Model file for the job. Use its own axes, mm. Face numbers are marked on the shaded views. A direction names the side the tool comes from. Round coordinates to 2 decimals unless told otherwise and drop trailing zeros. Write each loop counter-clockwise with the first axis right and the second up, starting at its lowest first coordinate (ties: lowest second). Pieces come first, ordered by that corner, then holes.
```python
from build123d import *

# Parameters (mm, degrees)
F0_W         = 50.8
F0_H         = 76.2
F1_DEPTH     = 6.35
F2_W         = 12.192
F2_H         = 25.4
F3_DEPTH     = 31.75
F5_D         = 12.7
F5_DEPTH     = 254
F5_TIP       = 3.8154649308
F6_R         = 12.69999
F7_T1_DEPTH  = 19.05001
F7_T3_DEPTH  = 76.2
F7_T5_DEPTH  = 38.1
F7_T7_DEPTH  = 38.1
F7_T9_DEPTH  = 2e-05
F7_T12_ANGLE = 90
F7_T14_ANGLE = 90
F7_T16_ANGLE = 90
F7_T18_ANGLE = 90
F7_T23_DEPTH = 31.75001
F7_T28_DEPTH = 38.1
F7_T35_DEPTH = 38.1
F7_T39_DEPTH = 31.75001
F7_T47_DEPTH = 38.1
F7_T51_DEPTH = 31.75001
F7_T59_DEPTH = 31.75001
F7_T64_DEPTH = 38.1


# Not quite as in the source:
# - a fillet or chamfer that OpenCascade refuses, or shapes differently, is made with other operations: its cross-section is extruded or revolved along the edge and cut away or added
# - a fillet or chamfer is up to 0.001 mm smaller than in the source, because OpenCascade refuses the exact size


with BuildPart() as f1:
    # F0 (on Top) → F1 (new body)
    with BuildSketch(Plane.XY):
        Rectangle(F0_W, F0_H)
    extrude(amount=F1_DEPTH)

    # F2 (on face) → F3 (join)
    with BuildSketch(Plane.XY.offset(6.35)):
        with Locations((-19.304, 0)):
            Rectangle(F2_W, F2_H)
        with Locations((19.304, 0)):
            Rectangle(F2_W, F2_H)
    extrude(amount=F3_DEPTH)

    # F5
    with Locations(Plane(origin=(-25.4, 0, 0), x_dir=(0, -1, 0), z_dir=(-1, 0, 0))):
        with Locations((0, 28.575)):
            Hole(F5_D / 2, depth=F5_DEPTH)
            with Locations((0, 0, -(F5_DEPTH + F5_TIP / 2))):  # 118° drill point
                Cone(0, F5_D / 2, F5_TIP, mode=Mode.SUBTRACT)

    # F6 (radius 12.7 in the source; OpenCascade refuses exactly that, so slightly less here)
    f6_edges = [f1.edges().sort_by_distance(p)[0] for p in [
        (19.304, 12.7, 38.1),
        (19.304, -12.7, 38.1),
        (-19.304, 12.7, 38.1),
        (-19.304, -12.7, 38.1),
    ]]
    fillet(f6_edges, radius=F6_R)

    # F7: fillet of radius 5.08 on 14 edges, made by hand

    # F7_s2 → F7_t1 (cut)
    with BuildSketch(Plane.XY.offset(6.35)):
        with BuildLine():
            ThreePointArc((-25.4, 7.62), (-23.9121024484, 11.2121024484), (-20.32, 12.7))
            Line((-20.32, 12.7), (-25.4, 12.7))
            Line((-25.4, 12.7), (-25.4, 7.62))
        make_face()
        with BuildLine():
            ThreePointArc((25.4, -7.62), (23.9121024484, -11.2121024484), (20.32, -12.7))
            Line((20.32, -12.7), (25.4, -12.7))
            Line((25.4, -12.7), (25.4, -7.62))
        make_face()
        with BuildLine():
            ThreePointArc((-25.4, -7.62), (-23.9121024484, -11.2121024484), (-20.32, -12.7))
            Line((-20.32, -12.7), (-25.4, -12.7))
            Line((-25.4, -12.7), (-25.4, -7.62))
        make_face()
        with BuildLine():
            ThreePointArc((25.4, 7.62), (23.9121024484, 11.2121024484), (20.32, 12.7))
            Line((20.32, 12.7), (25.4, 12.7))
            Line((25.4, 12.7), (25.4, 7.62))
        make_face()
    extrude(amount=F7_T1_DEPTH, mode=Mode.SUBTRACT)

    # F7_s4 → F7_t3 (cut)
    with BuildSketch(Plane.YZ.offset(-38.1)):
        with BuildLine():
            ThreePointArc((-33.02, 6.35), (-36.6121024484, 4.8621024484), (-38.1, 1.27))
            Line((-38.1, 1.27), (-38.1, 6.35))
            Line((-38.1, 6.35), (-33.02, 6.35))
        make_face()
        with BuildLine():
            ThreePointArc((33.02, 6.35), (36.6121024484, 4.8621024484), (38.1, 1.27))
            Line((38.1, 1.27), (38.1, 6.35))
            Line((38.1, 6.35), (33.02, 6.35))
        make_face()
    extrude(amount=F7_T3_DEPTH, mode=Mode.SUBTRACT)

    # F7_s6 → F7_t5 (cut)
    with BuildSketch(Plane.XZ.offset(12.7)):
        with BuildLine():
            ThreePointArc((20.32, 6.35), (23.9121024484, 4.8621024484), (25.4, 1.27))
            Line((25.4, 1.27), (25.4, 6.35))
            Line((25.4, 6.35), (20.32, 6.35))
        make_face()
        with BuildLine():
            ThreePointArc((-25.4, 1.27), (-23.9121024484, 4.8621024484), (-20.32, 6.35))
            Line((-20.32, 6.35), (-25.4, 6.35))
            Line((-25.4, 6.35), (-25.4, 1.27))
        make_face()
    extrude(amount=F7_T5_DEPTH, mode=Mode.SUBTRACT)

    # F7_s8 → F7_t7 (cut)
    with BuildSketch(Plane.XZ.offset(-50.8)):
        with BuildLine():
            ThreePointArc((20.32, 6.35), (23.9121024484, 4.8621024484), (25.4, 1.27))
            Line((25.4, 1.27), (25.4, 6.35))
            Line((25.4, 6.35), (20.32, 6.35))
        make_face()
        with BuildLine():
            ThreePointArc((-25.4, 1.27), (-23.9121024484, 4.8621024484), (-20.32, 6.35))
            Line((-20.32, 6.35), (-25.4, 6.35))
            Line((-25.4, 6.35), (-25.4, 1.27))
        make_face()
    extrude(amount=F7_T7_DEPTH, mode=Mode.SUBTRACT)

    # F7_s10 → F7_t9 (cut)
    with BuildSketch(Plane.XZ.offset(-1e-05)):
        with BuildLine():
            ThreePointArc((25.4, 33.02), (23.9121024484, 36.6121024484), (20.32, 38.1))
            Line((20.32, 38.1), (25.4, 38.1))
            Line((25.4, 38.1), (25.4, 33.02))
        make_face()
        with BuildLine():
            ThreePointArc((-25.4, 33.02), (-23.9121024484, 36.6121024484), (-20.32, 38.1))
            Line((-20.32, 38.1), (-25.4, 38.1))
            Line((-25.4, 38.1), (-25.4, 33.02))
        make_face()
    extrude(amount=F7_T9_DEPTH, mode=Mode.SUBTRACT)

    # F7_s11 → F7_t12 (revolve, cut)
    with BuildSketch(Plane.XY.offset(25.40001)):
        with BuildLine():
            ThreePointArc((-25.4, 7.62), (-23.9121024484, 11.2121024484), (-20.32, 12.7))
            Line((-20.32, 12.7), (-25.4, 12.7))
            Line((-25.4, 12.7), (-25.4, 7.62))
        make_face()
    revolve(axis=Axis((-25.4, 1e-05, 25.40001), (1, 0, 0)), revolution_arc=F7_T12_ANGLE, mode=Mode.SUBTRACT)

    # F7_s13 → F7_t14 (revolve, cut)
    with BuildSketch(Plane.XZ.offset(1e-05)):
        with BuildLine():
            ThreePointArc((-25.4, 33.02), (-23.9121024484, 36.6121024484), (-20.32, 38.1))
            Line((-20.32, 38.1), (-25.4, 38.1))
            Line((-25.4, 38.1), (-25.4, 33.02))
        make_face()
    revolve(axis=Axis((-25.4, -1e-05, 25.40001), (1, 0, 0)), revolution_arc=F7_T14_ANGLE, mode=Mode.SUBTRACT)

    # F7_s15 → F7_t16 (revolve, cut)
    with BuildSketch(Plane.XY.offset(25.40001)):
        with BuildLine():
            ThreePointArc((25.4, -7.62), (23.9121024484, -11.2121024484), (20.32, -12.7))
            Line((20.32, -12.7), (25.4, -12.7))
            Line((25.4, -12.7), (25.4, -7.62))
        make_face()
    revolve(axis=Axis((25.4, -1e-05, 25.40001), (-1, 0, 0)), revolution_arc=F7_T16_ANGLE, mode=Mode.SUBTRACT)

    # F7_s17 → F7_t18 (revolve, cut)
    with BuildSketch(Plane.XZ.offset(-1e-05)):
        with BuildLine():
            ThreePointArc((25.4, 33.02), (23.9121024484, 36.6121024484), (20.32, 38.1))
            Line((20.32, 38.1), (25.4, 38.1))
            Line((25.4, 38.1), (25.4, 33.02))
        make_face()
    revolve(axis=Axis((25.4, 1e-05, 25.40001), (-1, 0, 0)), revolution_arc=F7_T18_ANGLE, mode=Mode.SUBTRACT)


with BuildPart() as f7_tool21:
    # F7_s22 → F7_t23 (new body)
    with BuildSketch(Plane.XY.offset(-6.35)):
        with BuildLine():
            ThreePointArc((-25.4, 7.62), (-23.9121024484, 11.2121024484), (-20.32, 12.7))
            Line((-20.32, 12.7), (-25.4, 12.7))
            Line((-25.4, 12.7), (-25.4, 7.62))
        make_face()
    extrude(amount=F7_T23_DEPTH)

    split(bisect_by=Plane.XY.offset(6.35), keep=Keep.BOTTOM)

    split(bisect_by=Plane.XY, keep=Keep.TOP)


with BuildPart() as f7_tool26:
    # F7_s27 → F7_t28 (new body)
    with BuildSketch(Plane.XZ.offset(-38.1)):
        with BuildLine():
            ThreePointArc((-25.4, 1.27), (-23.9121024484, 4.8621024484), (-20.32, 6.35))
            Line((-20.32, 6.35), (-25.4, 6.35))
            Line((-25.4, 6.35), (-25.4, 1.27))
        make_face()
    extrude(amount=F7_T28_DEPTH)

    split(bisect_by=Plane.XZ.offset(-12.7), keep=Keep.TOP)


with BuildPart() as f7_tool21_1:
    add(f7_tool21.part)

    # F7_t30: intersect F7_tool26
    add(f7_tool26.part, mode=Mode.INTERSECT)


with BuildPart() as f1_1:
    add(f1.part)

    # F7_t19: cut F7_tool21
    add(f7_tool21_1.part, mode=Mode.SUBTRACT)


with BuildPart() as f7_tool33:
    # F7_s34 → F7_t35 (new body)
    with BuildSketch(Plane.XZ.offset(38.1)):
        with BuildLine():
            ThreePointArc((20.32, 6.35), (23.9121024484, 4.8621024484), (25.4, 1.27))
            Line((25.4, 1.27), (25.4, 6.35))
            Line((25.4, 6.35), (20.32, 6.35))
        make_face()
    extrude(amount=-F7_T35_DEPTH)

    split(bisect_by=Plane.XZ.offset(12.7), keep=Keep.BOTTOM)


with BuildPart() as f7_tool37:
    # F7_s38 → F7_t39 (new body)
    with BuildSketch(Plane.XY.offset(-6.35)):
        with BuildLine():
            ThreePointArc((25.4, -7.62), (23.9121024484, -11.2121024484), (20.32, -12.7))
            Line((20.32, -12.7), (25.4, -12.7))
            Line((25.4, -12.7), (25.4, -7.62))
        make_face()
    extrude(amount=F7_T39_DEPTH)

    split(bisect_by=Plane.XY.offset(6.35), keep=Keep.BOTTOM)

    split(bisect_by=Plane.XY, keep=Keep.TOP)


with BuildPart() as f7_tool33_1:
    add(f7_tool33.part)

    # F7_t42: intersect F7_tool37
    add(f7_tool37.part, mode=Mode.INTERSECT)


with BuildPart() as f1_2:
    add(f1_1.part)

    # F7_t31: cut F7_tool33
    add(f7_tool33_1.part, mode=Mode.SUBTRACT)


with BuildPart() as f7_tool45:
    # F7_s46 → F7_t47 (new body)
    with BuildSketch(Plane.XZ):
        with BuildLine():
            ThreePointArc((20.32, 6.35), (23.9121024484, 4.8621024484), (25.4, 1.27))
            Line((25.4, 1.27), (25.4, 6.35))
            Line((25.4, 6.35), (20.32, 6.35))
        make_face()
    extrude(amount=-F7_T47_DEPTH)

    split(bisect_by=Plane.XZ.offset(-12.7), keep=Keep.TOP)


with BuildPart() as f7_tool49:
    # F7_s50 → F7_t51 (new body)
    with BuildSketch(Plane.XY.offset(-6.35)):
        with BuildLine():
            ThreePointArc((25.4, 7.62), (23.9121024484, 11.2121024484), (20.32, 12.7))
            Line((20.32, 12.7), (25.4, 12.7))
            Line((25.4, 12.7), (25.4, 7.62))
        make_face()
    extrude(amount=F7_T51_DEPTH)

    split(bisect_by=Plane.XY.offset(6.35), keep=Keep.BOTTOM)

    split(bisect_by=Plane.XY, keep=Keep.TOP)


with BuildPart() as f7_tool45_1:
    add(f7_tool45.part)

    # F7_t54: intersect F7_tool49
    add(f7_tool49.part, mode=Mode.INTERSECT)


with BuildPart() as f1_3:
    add(f1_2.part)

    # F7_t43: cut F7_tool45
    add(f7_tool45_1.part, mode=Mode.SUBTRACT)


with BuildPart() as f7_tool57:
    # F7_s58 → F7_t59 (new body)
    with BuildSketch(Plane.XY.offset(-6.35)):
        with BuildLine():
            ThreePointArc((-25.4, -7.62), (-23.9121024484, -11.2121024484), (-20.32, -12.7))
            Line((-20.32, -12.7), (-25.4, -12.7))
            Line((-25.4, -12.7), (-25.4, -7.62))
        make_face()
    extrude(amount=F7_T59_DEPTH)

    split(bisect_by=Plane.XY.offset(6.35), keep=Keep.BOTTOM)

    split(bisect_by=Plane.XY, keep=Keep.TOP)


with BuildPart() as f7_tool62:
    # F7_s63 → F7_t64 (new body)
    with BuildSketch(Plane.XZ):
        with BuildLine():
            ThreePointArc((-25.4, 1.27), (-23.9121024484, 4.8621024484), (-20.32, 6.35))
            Line((-20.32, 6.35), (-25.4, 6.35))
            Line((-25.4, 6.35), (-25.4, 1.27))
        make_face()
    extrude(amount=F7_T64_DEPTH)

    split(bisect_by=Plane.XZ.offset(12.7), keep=Keep.BOTTOM)


with BuildPart() as f7_tool57_1:
    add(f7_tool57.part)

    # F7_t66: intersect F7_tool62
    add(f7_tool62.part, mode=Mode.INTERSECT)


with BuildPart() as f1_4:
    add(f1_3.part)

    # F7_t55: cut F7_tool57
    add(f7_tool57_1.part, mode=Mode.SUBTRACT)


solid = f1_4.part
```
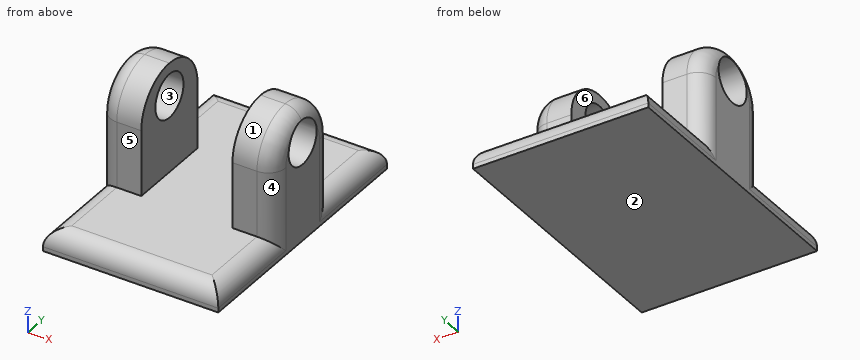
1) Wall check: probe 1 along Z at (x, y) = (19, 0) (3 decimals); probe 2 along X at (y, z) = (7, 7); probe 3 along Z at (x, y) = (11.5, -12). Give the ranges that are in metal, low to high.
2) Which spindle directions (+Z, -Z, +X, -X, +Y, -Y) get a long thin tool onto all of the face, cutting with end or side? Do the marked faces 4, 5 and 6. Say none if no direction does.
3) Cut at C-C on y = 20.5. List the corners of the cut face in (x, z), and give its area (3 significant figures).
4) Flat gauge pins, fed straight in: pin 1 Ø12 at (y, z) = (-24.5, 24) entering from -X; pin 2 Ø5.5 at (x, z) = (-15.5, 20.5) entering from +Y; pin 3 Ø3.5 at (x, z) = (15.5, 16) entering from -Y; pin 4 Ø2 at (x, y) = (-7, 27.5) entering from +Z. Where does each tip first touch, or does it go through?
5) Cut at A-A on z = 15.5. List the corners of the cut face in (x, y), and give its area (3 significant figures).
6) Cut at D-D on z = 24. List the corners of the cut face in (x, y).
7) Pull direction Y, two halves, no side cores. Call the marked faces 1, 2 and 3: released by +Y, released by -Y, zero draft, split by the parting line, or undercut.
Result sheet:
1. probe 1: z = 0 to 22.225, 34.925 to 38.1
1. probe 2: x = -25.4 to -13.21, 13.21 to 25.4
1. probe 3: z = 0 to 6.35
2. face 4: +Z, +X, -Y
2. face 5: +Z, +X, -X, -Y
2. face 6: +Z, +Y, -Y
3. outline: (-25.4, 0) - (25.4, 0) - (25.4, 1.27) arc R5.08 ccw to (20.32, 6.35) - (-20.32, 6.35) arc R5.08 ccw to (-25.4, 1.27) - close
3. area: 312 mm2
4. pin 1: passes through
4. pin 2: stops at y = 12.7
4. pin 3: stops at y = -12.7
4. pin 4: stops at z = 6.35
5. outline: (-25.4, -7.62) arc R5.08 ccw to (-20.32, -12.7) - (-13.21, -12.7) - (-13.21, 12.7) - (-20.32, 12.7) arc R5.08 ccw to (-25.4, 7.62) - close; (13.21, -12.7) - (20.32, -12.7) arc R5.08 ccw to (25.4, -7.62) - (25.4, 7.62) arc R5.08 ccw to (20.32, 12.7) - (13.21, 12.7) - close
5. area: 597 mm2
6. outline: (-25.4, -7.62) arc R5.08 ccw to (-20.32, -12.7) - (-13.21, -12.7) - (-13.21, -4.4) - (-25.4, -4.4) - close; (-25.4, 4.4) - (-13.21, 4.4) - (-13.21, 12.7) - (-20.32, 12.7) arc R5.08 ccw to (-25.4, 7.62) - close; (13.21, -12.7) - (20.32, -12.7) arc R5.08 ccw to (25.4, -7.62) - (25.4, -4.4) - (13.21, -4.4) - close; (13.21, 4.4) - (25.4, 4.4) - (25.4, 7.62) arc R5.08 ccw to (20.32, 12.7) - (13.21, 12.7) - close
7. face 1: released by -Y
7. face 2: zero draft
7. face 3: undercut
